Here's how the part is built. I have some questions about the finished solid (model axes, mm). A direction names the side the tool comes from. Coordinates: 2 decimals unless noted, no trailing zeros. Write each loop counter-clockwise with the first axis right and the second up, starting at its lowest first coordinate (ties: lowest second). Pieces come first, ordered by that corner, then holes.
```python
from build123d import *

# Parameters (mm, degrees)
SKETCH1_R                       = 5.334
BOSS_EXTRUDE1_DEPTH             = 19.05
F_4_0MM_DOWEL_HOLE2_D           = 4
F_4_0MM_DOWEL_HOLE2_DEPTH       = 9.525
F_4_0MM_DOWEL_HOLE2_TIP         = 1.201721238
F_3_16_0_1875_DOWEL_HOLE1_D     = 4.7625
F_3_16_0_1875_DOWEL_HOLE1_DEPTH = 9.525
F_3_16_0_1875_DOWEL_HOLE1_TIP   = 1.430799349
F_10_32_TAPPED_HOLE1_OUTLINE_R  = 2.0193
F_10_32_TAPPED_HOLE1_DEPTH      = 6


with BuildPart() as part:
    # Sketch1 → Boss-Extrude1 (new body)
    with BuildSketch(Plane(origin=(0, 0, 0), x_dir=(1, 0, 0), z_dir=(0, 1, 0))):
        with Locations(Location((0, 0, 0), (0, 0, 90))):
            Circle(SKETCH1_R)
    extrude(amount=BOSS_EXTRUDE1_DEPTH)

    # Ø4.0mm Dowel Hole2
    with Locations(Plane(origin=(0, 19.05, 0), x_dir=(1, 0, 0), z_dir=(0, 1, 0))):
        with Locations((0, 0)):
            Hole(F_4_0MM_DOWEL_HOLE2_D / 2, depth=F_4_0MM_DOWEL_HOLE2_DEPTH)
            with Locations((0, 0, -(F_4_0MM_DOWEL_HOLE2_DEPTH + F_4_0MM_DOWEL_HOLE2_TIP / 2))):  # 118° drill point
                Cone(0, F_4_0MM_DOWEL_HOLE2_D / 2, F_4_0MM_DOWEL_HOLE2_TIP, mode=Mode.SUBTRACT)

    # 3/16 (0.1875) Dowel Hole1
    with Locations(Plane(origin=(0, 0, 0), x_dir=(-1, 0, 0), z_dir=(0, -1, 0))):
        with Locations((0, 0)):
            Hole(F_3_16_0_1875_DOWEL_HOLE1_D / 2, depth=F_3_16_0_1875_DOWEL_HOLE1_DEPTH)
            with Locations((0, 0, -(F_3_16_0_1875_DOWEL_HOLE1_DEPTH + F_3_16_0_1875_DOWEL_HOLE1_TIP / 2))):  # 118° drill point
                Cone(0, F_3_16_0_1875_DOWEL_HOLE1_D / 2, F_3_16_0_1875_DOWEL_HOLE1_TIP, mode=Mode.SUBTRACT)

    # #10-32 Tapped Hole1: read off the stored shape, not the designer's step
    # #10-32 Tapped Hole1 outline → #10-32 Tapped Hole1 (cut)
    with BuildSketch(Plane.XY):
        with Locations((0, 3.429)):
            Circle(F_10_32_TAPPED_HOLE1_OUTLINE_R)
        with Locations((0, 15.621)):
            Circle(F_10_32_TAPPED_HOLE1_OUTLINE_R)
    extrude(amount=F_10_32_TAPPED_HOLE1_DEPTH, mode=Mode.SUBTRACT)


solid = part.part
```
1) We'd pull the mould along X, two halves only. Please class faces 1 (the face through (2.04, 9.39, -4.93)), 2 (the face through (-0.31, 4.83, -2.36)), 3 (the face through (1.1, 0, -2.3)): pulls with the +X half, pulls with the -X half, needs draft (parallel to the pull), parting line crosses it, or undercut.
Values follow:
face 1: parting line crosses it
face 2: undercut
face 3: needs draft
2) On a 3-axis mill with a long thin cutter (end or side, diameter ignored), from which of +Z, -Z, +X, -X, +Y, -Y can I reach the whole of each face in a straight line? I mean faces 4 (the face through (-2.017, 15.71, 3.224)), 5 (the face through (0, 14, -2)). Say none if no direction works.
Values follow:
face 4: +Z
face 5: +Y, -Y
3) I need wall thicknesses on probe 1 along Y at (x, z) = (0, 2.65); probe 2 along Y at (x, z) = (1.75, 4); probe 3 along X at (y, z) = (5.25, -0.25). Which ranges of each line are inside material? Lowest first, please.
Values follow:
probe 1: y = 0 to 1.41, 5.45 to 13.6, 17.64 to 19.05
probe 2: y = 0 to 2.42, 4.44 to 14.61, 16.63 to 19.05
probe 3: x = -5.33 to -2.37, 2.37 to 5.33
4) Imagine slicing it at C-C on y = 12. Please give me the cut outline in (x, z), then the cut area to 3 significant figures.
Values follow:
outline: circle Ø10.67 at (0, 0); hole circle Ø4 at (0, 0)
area: 76.8 mm2
5) Will these pins go through, and if not, where does the flat tip stop? pin 1 (4 mm diameter, centred on y = 11, z = -2.5, fed in from -X); pin 2 (1.5 mm diameter, centred on x = 4, y = 12, fed in from +Z); pin 3 (1.5 mm diameter, centred on x = 0, z = -1.5, fed in from -Y).
Values follow:
pin 1: stops at x = -5.31
pin 2: stops at z = 4.23
pin 3: stops at y = 9.6
6) Imagine slicing it at B-B on y = 8.5. Please give me the cut outline in (x, z).
Values follow:
outline: circle Ø10.67 at (0, 0); hole circle Ø4.76 at (0, 0)
7) Imagine slicing it at D-D on x = -1.75. Count the separate pieces of the cut face and the enclosed holes in it, then the cut area to 3 significant figures.
Values follow:
separate pieces: 4
enclosed holes: 0
area: 128 mm2
8) Imagine slicing it at A-A on x = 0. Please give me the cut outline in (y, z) (3 decimals).
Values follow:
outline: (0, -5.334) - (19.05, -5.334) - (19.05, -2) - (9.754, -2) - (9.525, -2.381) - (0, -2.381) - close; (0, 2.381) - (1.41, 2.381) - (1.41, 5.334) - (0, 5.334) - close; (5.448, 2.381) - (9.525, 2.381) - (9.754, 2) - (13.602, 2) - (13.602, 5.334) - (5.448, 5.334) - close; (17.64, 2) - (19.05, 2) - (19.05, 5.334) - (17.64, 5.334) - close
